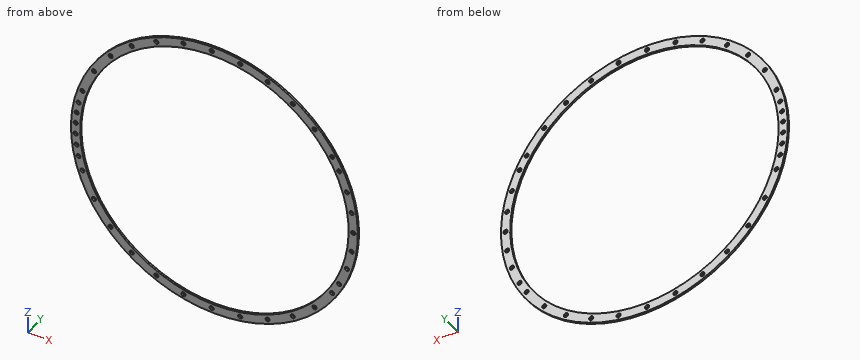
from build123d import *

# Parameters (mm, degrees)
SKETCH1_W          = 7
SKETCH1_H          = 1.5
SKETCH3_R          = 1.6
CUT_EXTRUDE2_DEPTH = 155.156576246


with BuildPart() as part:
    # Sketch1 → Revolve1 (revolve)
    with BuildSketch(Plane.XY, mode=Mode.PRIVATE) as revolve1_sk:
        with Locations((-105.5, 3.925)):
            Rectangle(SKETCH1_W, SKETCH1_H)
    revolve(revolve1_sk.sketch.rotate(Axis((0, -200069.047495165, 0), (0, 1, 0)), 270), axis=Axis((0, -200069.047495165, 0), (0, 1, 0)))

    # Sketch3 → Cut-Extrude2 (cut, through all)
    with BuildSketch(Plane(origin=(0, 4.675, 0), x_dir=(1, 0, 0), z_dir=(0, 1, 0))):
        with Locations(Location((-103.194571877, -21.934683381, 0), (0, 0, 270))):
            Circle(SKETCH3_R)
        with Locations(Location((-105.407458575, -4.417881468, 0), (0, 0, 270))):
            Circle(SKETCH3_R)
        with Locations(Location((-104.668100989, -13.222656141, 0), (0, 0, 270))):
            Circle(SKETCH3_R)
        with Locations(Location((-100.336462469, 32.601292907, 0), (0, 0, 270))):
            Circle(SKETCH3_R)
        with Locations(Location((104.295371407, 15.897342642, 0), (0, 0, 270))):
            Circle(SKETCH3_R)
        with Locations(Location((100.708995202, 31.43164465, 0), (0, 0, 270))):
            Circle(SKETCH3_R)
        with Locations(Location((94.822771885, 46.248155986, 0), (0, 0, 270))):
            Circle(SKETCH3_R)
        with Locations(Location((-103.194571877, 21.934683381, 0), (0, 0, 270))):
            Circle(SKETCH3_R)
        with Locations(Location((-104.668100989, 13.222656141, 0), (0, 0, 270))):
            Circle(SKETCH3_R)
        with Locations(Location((-105.407458575, 4.417881468, 0), (0, 0, 270))):
            Circle(SKETCH3_R)
        with Locations(Location((89.469074145, -55.906482377, 0), (0, 0, 270))):
            Circle(SKETCH3_R)
        with Locations(Location((-44.130594647, 95.826617472, 0), (0, 0, 270))):
            Circle(SKETCH3_R)
        with Locations(Location((-62.82106423, 84.757087545, 0), (0, 0, 270))):
            Circle(SKETCH3_R)
        with Locations(Location((-78.848228037, 70.094271773, 0), (0, 0, 270))):
            Circle(SKETCH3_R)
        with Locations(Location((-91.532612735, 52.45980181, 0), (0, 0, 270))):
            Circle(SKETCH3_R)
        with Locations(Location((94.822771885, -46.248155986, 0), (0, 0, 270))):
            Circle(SKETCH3_R)
        with Locations(Location((100.708995202, -31.43164465, 0), (0, 0, 270))):
            Circle(SKETCH3_R)
        with Locations(Location((104.295371407, -15.897342642, 0), (0, 0, 270))):
            Circle(SKETCH3_R)
        with Locations(Location((105.5, 0, 0), (0, 0, 270))):
            Circle(SKETCH3_R)
        with Locations(Location((76.122528254, -73.04526468, 0), (0, 0, 270))):
            Circle(SKETCH3_R)
        with Locations(Location((89.469074145, 55.906482377, 0), (0, 0, 270))):
            Circle(SKETCH3_R)
        with Locations(Location((76.122528254, 73.04526468, 0), (0, 0, 270))):
            Circle(SKETCH3_R)
        with Locations(Location((59.54875959, 87.08728513, 0), (0, 0, 270))):
            Circle(SKETCH3_R)
        with Locations(Location((40.450414858, 97.437230758, 0), (0, 0, 270))):
            Circle(SKETCH3_R)
        with Locations(Location((19.637170436, 103.656314507, 0), (0, 0, 270))):
            Circle(SKETCH3_R)
        with Locations(Location((-2.008593938, 105.480877653, 0), (0, 0, 270))):
            Circle(SKETCH3_R)
        with Locations(Location((-23.569203757, 102.833567643, 0), (0, 0, 270))):
            Circle(SKETCH3_R)
        with Locations(Location((-91.532612735, -52.45980181, 0), (0, 0, 270))):
            Circle(SKETCH3_R)
        with Locations(Location((-62.82106423, -84.757087545, 0), (0, 0, 270))):
            Circle(SKETCH3_R)
        with Locations(Location((-44.130594647, -95.826617472, 0), (0, 0, 270))):
            Circle(SKETCH3_R)
        with Locations(Location((-23.569203757, -102.833567643, 0), (0, 0, 270))):
            Circle(SKETCH3_R)
        with Locations(Location((-2.008593938, -105.480877653, 0), (0, 0, 270))):
            Circle(SKETCH3_R)
        with Locations(Location((19.637170436, -103.656314507, 0), (0, 0, 270))):
            Circle(SKETCH3_R)
        with Locations(Location((40.450414858, -97.437230758, 0), (0, 0, 270))):
            Circle(SKETCH3_R)
        with Locations(Location((59.54875959, -87.08728513, 0), (0, 0, 270))):
            Circle(SKETCH3_R)
        with Locations(Location((-78.848228037, -70.094271773, 0), (0, 0, 270))):
            Circle(SKETCH3_R)
        with Locations(Location((-100.336462469, -32.601292907, 0), (0, 0, 270))):
            Circle(SKETCH3_R)
    extrude(amount=-CUT_EXTRUDE2_DEPTH, mode=Mode.SUBTRACT)


solid = part.part
Geometry check sheet. Reference: the model listing, model coordinates, mm. Round coordinates to 2 decimals unless told otherwise and drop trailing zeros. Loops run counter-clockwise (first coordinate to the right, second up) from the corner with the lowest first, then second, coordinate; pieces in that order, holes last. Notation, with made-up numbers: (-30.5, 62.25) - (28.5, 62.25) arc R23 ccw to (28.5, 76.25) - close; hole circle Ø10 at (20.5, -11.75). An arc over 180 degrees is marked (long way). One line per question, with ' | ' between items. Start each with the question number.
1. Cross-section at A-A on z = 41. Record the cut outline in (x, y) (3 decimals).
2. Scan lines: line 1 (X direction, y = 4.2, z = 15); line 2 (Z direction, x = 58.5, y = 4.5); line 3 (X direction, y = 3.65, z = 52). Record each from-to range of solid material in increasing order. Write a range as [from, to].
3. Cross-section at C-C on y = 3.6. State how many separate pieces and enclosed holes the cut face has, then the cut area to 3 significant figures.
4. Depth check by flat-ended pin: pin 1 (3.5 mm diameter, centred on x = -44.13, z = -95.83, fed in from -Y) (3 decimals). Enter the tip coordinate at first touch or a pass-through.
5. Cross-section at B-B on x = -70. Record the cut outline in (y, z) (3 decimals), then the cut area to 3 significant figures.
Taken from the geometry:
1) outline: (-100.995, 3.175) - (-93.397, 3.175) - (-93.397, 4.675) - (-100.995, 4.675) - close; (93.397, 3.175) - (100.995, 3.175) - (100.995, 4.675) - (93.397, 4.675) - close
2) line 1: [-107.96, -100.89], [100.89, 102.97], [105.62, 107.96] | line 2: [-91.97, -88.3], [-85.88, -83.56], [83.56, 85.88], [88.3, 91.97] | line 3: [-95.8, -93.07], [-90, -87.75], [87.75, 95.8]
3) separate pieces: 1 | enclosed holes: 38 | area: 4,340 mm²
4) pin 1: y = 3.175
5) outline: (3.175, -83.552) - (4.675, -83.552) - (4.675, -74.189) - (3.175, -74.189) - close; (3.175, 74.189) - (4.675, 74.189) - (4.675, 83.552) - (3.175, 83.552) - close | area: 28.1 mm²
